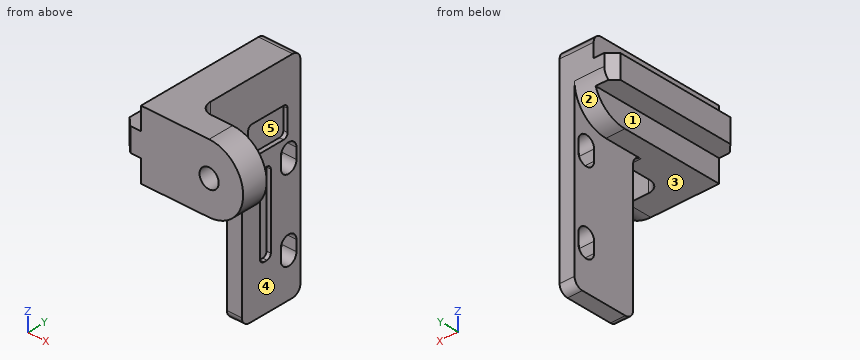
```python
from build123d import *

# Parameters (mm, degrees)
BOSS_EXTRUDE1_DEPTH = 8
SKETCH2_W           = 5.5
SKETCH2_H           = 32
BOSS_EXTRUDE2_DEPTH = 4.5
CUT_EXTRUDE2_DEPTH  = 1
SKETCH5_W           = 4.5
SKETCH5_H           = 34
CUT_EXTRUDE3_DEPTH  = 53.351043088
FILLET4_R           = 2
CHAMFER1_SIZE       = 2
SKETCH6_R           = 2.25
BOSS_EXTRUDE3_DEPTH = 6
FILLET5_R           = 8
FILLET6_R           = 3


with BuildPart() as part:
    # Sketch1 → Boss-Extrude1 (new body)
    with BuildSketch(Plane(origin=(0, 0, 0), x_dir=(0, 0, -1), z_dir=(1, 0, 0))):
        Polygon((-32.846556001, 14.959797641), (-32.846556001, -2.08853598), (-48.846556001, -2.08853598), (-48.846556001, 29.91146402), (1.153443999, 29.91146402), (1.153443999, 14.959797641), align=None)
        with BuildLine():
            Line((-29.23609438, 28.91146402), (-26.73609438, 28.91146402))
            ThreePointArc((-26.73609438, 28.91146402), (-24.73609438, 26.91146402), (-26.73609438, 24.91146402))
            Line((-26.73609438, 24.91146402), (-29.23609438, 24.91146402))
            ThreePointArc((-29.23609438, 24.91146402), (-31.23609438, 26.91146402), (-29.23609438, 28.91146402))
        make_face(mode=Mode.SUBTRACT)
        with BuildLine():
            Line((-10.346556001, 28.91146402), (-7.846556001, 28.91146402))
            ThreePointArc((-7.846556001, 28.91146402), (-5.846556001, 26.91146402), (-7.846556001, 24.91146402))
            Line((-7.846556001, 24.91146402), (-10.346556001, 24.91146402))
            ThreePointArc((-10.346556001, 24.91146402), (-12.346556001, 26.91146402), (-10.346556001, 28.91146402))
        make_face(mode=Mode.SUBTRACT)
    extrude(amount=BOSS_EXTRUDE1_DEPTH)

    # Sketch2 → Boss-Extrude2 (add)
    with BuildSketch(Plane.ZY):
        with Locations((40.846556001, 13.91146402)):
            Rectangle(SKETCH2_W, SKETCH2_H)
    extrude(amount=BOSS_EXTRUDE2_DEPTH)

    # Sketch4 → Cut-Extrude2 (cut)
    with BuildSketch(Plane(origin=(8, 0, 0), x_dir=(0, 0, -1), z_dir=(1, 0, 0))):
        with BuildLine():
            Line((-33.306145699, 26.647879309), (-38.295392652, 26.647879309))
            ThreePointArc((-38.295392652, 26.647879309), (-39.002499434, 26.354986091), (-39.295392652, 25.647879309))
            Line((-39.295392652, 25.647879309), (-39.295392652, 17.565584617))
            ThreePointArc((-39.295392652, 17.565584617), (-39.002499434, 16.858477836), (-38.295392652, 16.565584617))
            Line((-38.295392652, 16.565584617), (-33.306145699, 16.565584617))
            ThreePointArc((-33.306145699, 16.565584617), (-32.599038918, 16.858477836), (-32.306145699, 17.565584617))
            Line((-32.306145699, 17.565584617), (-32.306145699, 25.647879309))
            ThreePointArc((-32.306145699, 25.647879309), (-32.599038918, 26.354986091), (-33.306145699, 26.647879309))
        make_face()
        with BuildLine():
            Line((-27.806359761, 22.368339675), (-10.62033731, 22.368339675))
            ThreePointArc((-10.62033731, 22.368339675), (-9.913230529, 22.075446457), (-9.62033731, 21.368339675))
            Line((-9.62033731, 21.368339675), (-9.62033731, 20.617921417))
            ThreePointArc((-9.62033731, 20.617921417), (-9.913230529, 19.910814636), (-10.62033731, 19.617921417))
            Line((-10.62033731, 19.617921417), (-27.806359761, 19.617921417))
            ThreePointArc((-27.806359761, 19.617921417), (-28.513466542, 19.910814636), (-28.806359761, 20.617921417))
            Line((-28.806359761, 20.617921417), (-28.806359761, 21.368339675))
            ThreePointArc((-28.806359761, 21.368339675), (-28.513466542, 22.075446457), (-27.806359761, 22.368339675))
        make_face()
    extrude(amount=-CUT_EXTRUDE2_DEPTH, mode=Mode.SUBTRACT)

    # Sketch5 → Cut-Extrude3 (cut, through all)
    with BuildSketch(Plane.XZ.offset(-14.959797641)):
        with Locations((2.25, 15.846556001)):
            Rectangle(SKETCH5_W, SKETCH5_H)
    extrude(amount=-CUT_EXTRUDE3_DEPTH, mode=Mode.SUBTRACT)

    # Fillet4
    fillet4_edges = [part.edges().sort_by_distance(p)[0] for p in [
        (6.25, 29.91146402, -1.153443999),
        (6.25, 14.959797641, -1.153443999),
        (6.25, 14.959797641, 32.846556001),
        (4, 29.91146402, 48.846556001),
    ]]
    fillet(fillet4_edges, radius=FILLET4_R)

    # Chamfer1
    chamfer1_edges = [part.edges().sort_by_distance(p)[0] for p in [
        (-4.5, -2.08853598, 40.846556001),
        (-4.5, 29.91146402, 40.846556001),
    ]]
    chamfer(chamfer1_edges, length=CHAMFER1_SIZE)

    # Sketch6 → Boss-Extrude3 (add)
    with BuildSketch(Plane.XZ.offset(2.08853598)):
        with BuildLine():
            Line((8, 48.846556001), (16, 48.846556001))
            ThreePointArc((16, 48.846556001), (24, 40.846556001), (16, 32.846556001))
            Line((16, 32.846556001), (8, 32.846556001))
            Line((8, 32.846556001), (8, 48.846556001))
        make_face()
        with Locations(Location((16, 40.846556001, 0), (0, 0, 270))):
            Circle(SKETCH6_R, mode=Mode.SUBTRACT)
    extrude(amount=-BOSS_EXTRUDE3_DEPTH)

    # Fillet5
    fillet5_edges = [part.edges().sort_by_distance(p)[0] for p in [
        (2.25, 29.91146402, 32.846556001),
    ]]
    fillet(fillet5_edges, radius=FILLET5_R)

    # Fillet6
    fillet6_edges = [part.edges().sort_by_distance(p)[0] for p in [
        (8, 3.91146402, 40.846556001),
    ]]
    fillet(fillet6_edges, radius=FILLET6_R)


solid = part.part
```
Build history of the part. All positions in model axes, mm. Face numbers are marked on the shaded views. A direction names the side the tool comes from. Round coordinates to 2 decimals unless told otherwise and drop trailing zeros. Order: outer loops, then holes, each group sorted by start corner. A loop starts at its lowest first (then second) coordinate and runs counter-clockwise, first axis right, second up. Notation, with made-up numbers: (18.25, -29.75) -> (74.25, -29.75) arc R12 cw to (74.25, -19.75) -> close; hole circle Ø8 at (-7, -19.75). An arc over 180 degrees is marked (long way). Answer in a Markdown table with one row per item.
1) Wall check: L1, parallel to X at y = 1.5, z = 41; L2, parallel to X at y = 20, z = 34.5; L3, parallel to X at y = 17.5, z = 24.5. Give the ranges that are in metal, low to high.
Values:
| item | result |
|---|---|
| L1 | -4.5 to 13.76, 18.24 to 24 |
| L2 | 0 to 7 |
| L3 | 4.5 to 8 |
2) Band-saw the part on A-A on z = 20. Give the cut face in (x, y).
Values:
| item | result |
|---|---|
| outline | (4.5, 14.96) -> (8, 14.96) -> (8, 19.62) -> (7, 19.62) -> (7, 22.37) -> (8, 22.37) -> (8, 29.91) -> (4.5, 29.91) -> close |
3) Pin check, flat tips, straight feed: P1, Ø8.5, axis at y = 21, z = 24.5, coming from the -X side; P2, Ø18.5, axis at y = 23.5, z = 12, coming from the +X side; P3, Ø2.5, axis at y = 10, z = 47, coming from the -X side. Stop position of each tip, or through.
Values:
| item | result |
|---|---|
| P1 | x = 4.5 |
| P2 | x = 8 |
| P3 | x = 0 |
4) Which spindle directions (+Z, -Z, +X, -X, +Y, -Y) get a long thin tool onto all of the face, cutting with end or side? Do the marked faces 1, 2, 3, 4 and 5. Say none if no direction does.
Values:
| item | result |
|---|---|
| face 1 | -Z, -X, +Y, -Y |
| face 2 | -Z, -X, +Y |
| face 3 | -Z, -X, -Y |
| face 4 | +Z, -Z, +X, +Y |
| face 5 | +X |
5) Band-saw the part on D-D on y = 24. Give the cut face in (x, z), and give its area (3 significant figures).
Values:
| item | result |
|---|---|
| outline | (-4.5, 38.1) -> (0, 38.1) -> (0, 33.12) -> (4.5, 33.12) -> (4.5, -1.15) -> (8, -1.15) -> (8, 32.31) -> (7, 32.31) -> (7, 39.3) -> (8, 39.3) -> (8, 48.85) -> (0, 48.85) -> (0, 43.6) -> (-4.5, 43.6) -> close |
| area | 264 mm2 |
6) Band-saw the part on B-B on z = 6.5. Give the cut face in (x, y), and give its area (3 significant figures).
Values:
| item | result |
|---|---|
| outline | (4.5, 14.96) -> (8, 14.96) -> (8, 25.43) -> (4.5, 25.43) -> close; (4.5, 28.39) -> (8, 28.39) -> (8, 29.91) -> (4.5, 29.91) -> close |
| area | 42.0 mm2 |
7) Band-saw the part on C-C on x = 12.25. Give the cut face in (y, z), and give its area (3 significant figures).
Values:
| item | result |
|---|---|
| outline | (-2.09, 32.85) -> (3.91, 32.85) -> (3.91, 48.85) -> (-2.09, 48.85) -> close |
| area | 96.0 mm2 |
